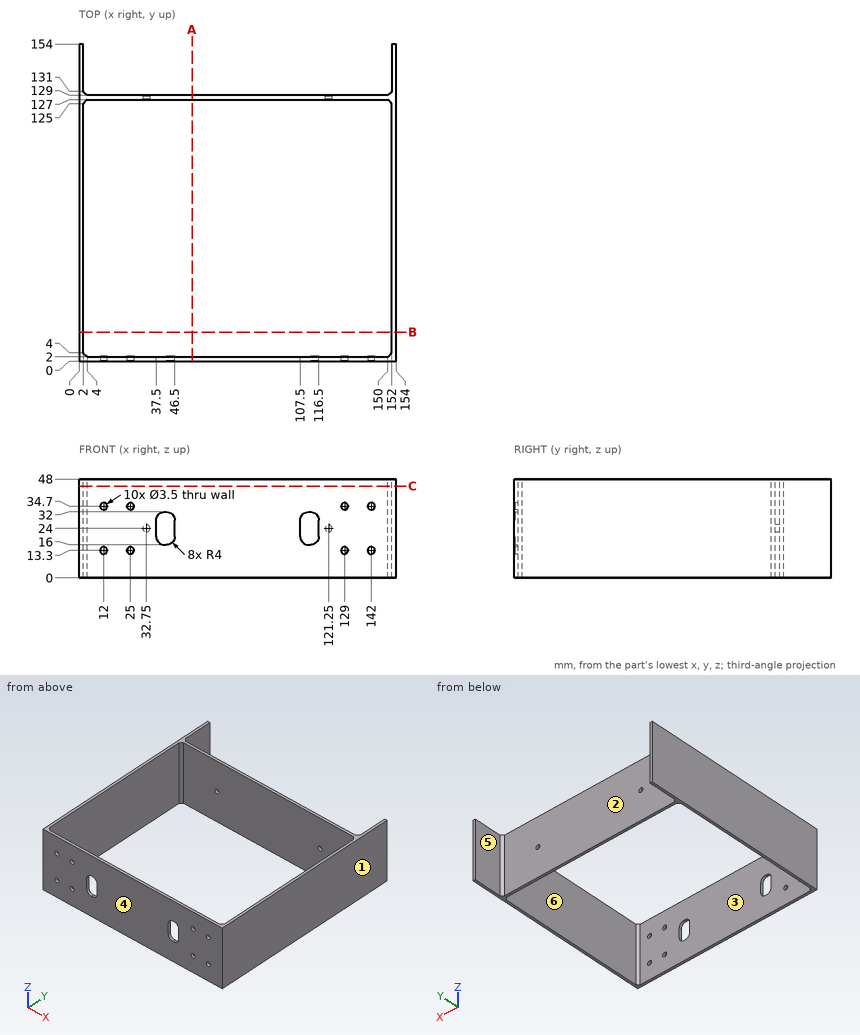
Job drawing, mm, ordinate dimensions from the low corner. One solid piece. A direction names the side the tool comes from. Coordinates: 2 decimals unless noted, no trailing zeros. Write each loop counter-clockwise with the first axis right and the second up, starting at its lowest first coordinate (ties: lowest second). Pieces come first, ordered by that corner, then holes. Notation, with made-up numbers: M 60,-21.5 L 82,-21.5 A17 cw 82,-2.5 Z; hole C -20.5,89 d3. An arc over 180 degrees is marked long. Answer as a JSON object with one key per item and string values. Group by question number.
1) Saw through at B-B (y = 14). Write the cut outline in (x, z), plus the area to 3 significant figures.
2) Wall check: line 1 (Z direction, x = 25, y = 0.5); line 2 (X direction, y = 48, z = 22.5); line 3 (Y direction, x = 35, z = 31). Give the ranges that are in metal, low to high. Write a range as from..to.
3) Mould opens along Y. For the marked faces 1, 2 and 3 say: +Y half, -Y half, draft (parallel to the pull), parting line (faces both ways), or undercut.
4) Saw through at A-A (x = 55). Write the cut outline in (y, z), plus the area to 3 significant figures.
5) Tool access for the marked faces 4, 5 and 6: list every direction of +Z, -Z, +X, -X, +Y, -Y with a clear straight run to the whole face (end or side of a thin tool).
6) Pin check, flat tip, straight feed: pin 1 Ø5.5 at (x, z) = (129, 13.3) entering from +Y. Stop position of the tip, or through.
7) Saw through at C-C (z = 44.5). Write the cut outline in (x, y).
Values follow:
{
 "1": {"outline": "M 0,0 L 2,0 L 2,48 L 0,48 Z; M 152,0 L 154,0 L 154,48 L 152,48 Z", "area": "192 mm2"},
 "2": {"line 1": "z = 0..11.55, 15.05..32.95, 36.45..48", "line 2": "x = 0..2, 152..154", "line 3": "y = 0..2, 127..129"},
 "3": {"face 1": "draft", "face 2": "+Y half", "face 3": "undercut"},
 "4": {"outline": "M 0,0 L 2,0 L 2,48 L 0,48 Z; M 127,0 L 129,0 L 129,48 L 127,48 Z", "area": "192 mm2"},
 "5": {"face 4": "+Z, -Z, +X, -X, -Y", "face 5": "+Z, -Z, +Y", "face 6": "+Z, -Z"},
 "6": {"pin 1": "stops at y = 129"},
 "7": {"outline": "M 0,0 L 154,0 L 154,154 L 152,154 L 152,131 L 150,129 L 4,129 L 2,131 L 2,154 L 0,154 Z; hole M 2,4 L 4,2 L 150,2 L 152,4 L 152,125 L 150,127 L 4,127 L 2,125 Z"}
}
